```python
from build123d import *

# Parameters (mm, degrees)
SKETCH_1_W          = 29.5
SKETCH_1_H          = 29.5
EXTRUDE_1_DEPTH     = 15
SKETCH_4_R          = 5.854360827
CUT_EXTRUDE_1_DEPTH = 1
SKETCH_5_W          = 8.438163648
SKETCH_5_H          = 4.320992013
SKETCH_5_W_2        = 9.049624782
SKETCH_5_H_2        = 3.485328464
CUT_EXTRUDE_2_DEPTH = 1


with BuildPart() as part:
    # 草图1 → 凸台-拉伸1 (new body)
    with BuildSketch(Plane(origin=(0, 0, 0), x_dir=(1, 0, 0), z_dir=(0, 1, 0))):
        Rectangle(SKETCH_1_W, SKETCH_1_H)
    extrude(amount=EXTRUDE_1_DEPTH)

    # 草图4 → 切除-拉伸1 (cut)
    with BuildSketch(Plane(origin=(0, 15, 0), x_dir=(1, 0, 0), z_dir=(0, 1, 0))):
        with Locations(Location((-6.828709963, 4.814266748, 0), (0, 0, 270))):
            Circle(SKETCH_4_R)
        with BuildLine():
            Line((5.371174923, 7.377688131), (8.366864515, 7.377688131))
            ThreePointArc((8.366864515, 7.377688131), (10.991875344, 4.752677302), (8.366864515, 2.127666472))
            Line((8.366864515, 2.127666472), (5.371174923, 2.127666472))
            ThreePointArc((5.371174923, 2.127666472), (2.746164094, 4.752677302), (5.371174923, 7.377688131))
        make_face()
    extrude(amount=-CUT_EXTRUDE_1_DEPTH, mode=Mode.SUBTRACT)

    # 草图5 → 切除-拉伸2 (cut)
    with BuildSketch(Plane.XY.offset(14.75)):
        with Locations((5.778081635, 6.579139216)):
            Rectangle(SKETCH_5_W, SKETCH_5_H)
        with Locations((-5.268982852, 6.161307442)):
            Rectangle(SKETCH_5_W_2, SKETCH_5_H_2)
    extrude(amount=-CUT_EXTRUDE_2_DEPTH, mode=Mode.SUBTRACT)


solid = part.part
```
Model file for the job. Use its own axes, mm. A direction names the side the tool comes from. Round coordinates to 2 decimals unless told otherwise and drop trailing zeros. Write each loop counter-clockwise with the first axis right and the second up, starting at its lowest first coordinate (ties: lowest second). Pieces come first, ordered by that corner, then holes. Notation, with made-up numbers: M 56,30 L 104,30 A32 cw 104,63 Z; hole C 2.5,9.5 d8. An arc over 180 degrees is marked long. Put each result on its own line as item: value.
Item 1: Cut at A-A (z = -1). List the corners of the cut face in (x, y), and give its area (3 significant figures).
Responses:
outline: M -14.75,0 L 14.75,0 L 14.75,15 L -2.39,15 L -2.39,14 L -11.27,14 L -11.27,15 L -14.75,15 Z
area: 434 mm²
Item 2: Flat gauge pins, fed straight in: P1, Ø1.7, axis at x = -5, y = 6.5, coming from the +Z side; P2, Ø7, axis at x = -6.83, z = -4.81, coming from the +Y side. Where does each tip first touch, or does it go through?
Responses:
P1: z = 13.75
P2: y = 14
Item 3: Mould opens along X. For faces 4 (the flat face through (6.8, 14.5, -7.378)), 5 (the flat face through (-14.75, 7, 0)), 6 (the flat face through (0, 7, 14.75)) say: +X half, -X half, draft (parallel to the pull), parting line (faces both ways), or undercut.
Responses:
face 4: undercut
face 5: -X half
face 6: draft
Item 4: Cut at C-C (x = -10.75). List the corners of the cut face in (y, z), and give its area (3 significant figures).
Responses:
outline: M 0,-14.75 L 15,-14.75 L 15,-9.16 L 14,-9.16 L 14,-0.47 L 15,-0.47 L 15,14.75 L 0,14.75 Z
area: 434 mm²
Item 5: Cut at B-B (y = 5). List the corners of the cut face in (x, z), and give its area (3 significant figures).
Responses:
outline: M -14.75,-14.75 L 14.75,-14.75 L 14.75,14.75 L 10,14.75 L 10,13.75 L 1.56,13.75 L 1.56,14.75 L -0.74,14.75 L -0.74,13.75 L -9.79,13.75 L -9.79,14.75 L -14.75,14.75 Z
area: 853 mm²
Item 6: Tool access for faces 1 (the flat face through (6, 8.74, 14)), 2 (the flat face through (14.75, 7, 0)), 3 (the flat face through (6.9, 14.5, -2.128)): list every direction of +Z, -Z, +X, -X, +Y, -Y with a clear straight run to the whole face (end or side of a thin tool).
Responses:
face 1: +Z
face 2: +Z, -Z, +X, +Y, -Y
face 3: +Y
Item 7: Probe L1, parallel to Y at x = 8.5, z = -4; L2, parallel to Z at x = -8.5, y = 5. List the from-to ranges inside material, lowest first. Write a range as from..to.
Responses:
L1: 0..14
L2: -14.75..13.75
Item 8: Cut at D-D (x = -5.25). List the corners of the cut face in (y, z).
Responses:
outline: M 0,-14.75 L 15,-14.75 L 15,-10.45 L 14,-10.45 L 14,0.82 L 15,0.82 L 15,14.75 L 7.9,14.75 L 7.9,13.75 L 4.42,13.75 L 4.42,14.75 L 0,14.75 Z
